from build123d import *

# Parameters (mm, degrees)
F1_DEPTH = 38.1
F2_R     = 10.16
F3_DEPTH = 35.56
F5_DEPTH = 19.05
F7_DEPTH = 18.796


with BuildPart() as f1:
    # F0 (on Top) → F1 (new body)
    with BuildSketch(Plane.XY):
        Polygon((-12.0983748909, -20.955), (12.0983748909, -20.955), (24.1967497817, 0), (12.0983748909, 20.955), (-12.0983748909, 20.955), (-24.1967497817, 0), align=None)
    extrude(amount=F1_DEPTH)

    # F2 (on face) → F3 (cut)
    with BuildSketch(Plane.XY.offset(38.1)):
        with Locations((-5.499261314, 9.525)):
            Circle(F2_R)
        with Locations((5.499261314, -9.525)):
            Circle(F2_R)
    extrude(amount=-F3_DEPTH, mode=Mode.SUBTRACT)

    # F4 (on face) → F5 (cut)
    with BuildSketch(Plane(origin=(0, 0, 0), x_dir=(1, 0, 0), z_dir=(0, 0, -1))):
        Polygon((-15.9478578107, 9.2075), (-18.1475623363, 10.4775), (-19.4175623363, 8.2777954744), (-17.8528578107, 5.9079432116), align=None)
        Polygon((-16.8775623363, 12.6772045256), (-18.1475623363, 10.4775), (-15.9478578107, 9.2075), (-14.0428578107, 12.5070567884), align=None)
    extrude(amount=-F5_DEPTH, mode=Mode.SUBTRACT)

    # F6 (on face) → F7 (join)
    with BuildSketch(Plane(origin=(0, 0, 0), x_dir=(1, 0, 0), z_dir=(0, 0, -1))):
        Polygon((-2.286, 20.955), (0, 20.955), (0, 23.241), (-3.429, 23.241), align=None)
        Polygon((0, 23.241), (0, 20.955), (2.286, 20.955), (3.429, 23.241), align=None)
    extrude(amount=-F7_DEPTH)


solid = f1.part
Check sheet for the modelled part. Datum: model origin and axes. Units: mm. A direction names the side the tool comes from. Coordinates: 2 decimals unless noted, no trailing zeros. Loops run counter-clockwise (first coordinate to the right, second up) from the corner with the lowest first, then second, coordinate; pieces in that order, holes last. Notation, with made-up numbers: (41.5, 69.5) -> (65.5, 69.5) arc R7 ccw to (65.5, 74.5) -> close; hole circle Ø3 at (12, 59). An arc over 180 degrees is marked (long way). Answer in a Markdown table with one row per item.
1. Access from +Z, -Z, +X, -X, +Y, -Y to the whole of each face (thin tool, end or side, straight path). Record for faces 5 (the face through (2.85, -22.08, 9.27)), 6 (the face through (15.2, -6.5, 20.6)), 7 (the face through (-17, -10, 19.05)), 8 (the face through (-18.646, -7.109, 9.392)).
Check values:
| item | result |
|---|---|
| face 5 | +Z, -Z, +X |
| face 6 | +Z |
| face 7 | -Z |
| face 8 | -Z, -Y |
2. Release check for a two-part mould opening along Y. For faces 1 (the face through (0, -1, 0)), 2 (the face through (0, -23.241, 9)), 3 (the face through (5, -9, 2.54)), 4 (the face through (18.232, 10.331, 18.783)) record: released by +Y, released by -Y, zero draft, split by the parting line, or undercut.
Check values:
| item | result |
|---|---|
| face 1 | zero draft |
| face 2 | released by -Y |
| face 3 | undercut |
| face 4 | released by +Y |
3. Sectioned sample at D-D, the plane z = 21.5. Record the boundary of the cut face in (x, y) (3 decimals).
Check values:
| item | result |
|---|---|
| outline | (-24.197, 0) -> (-12.098, -20.955) -> (12.098, -20.955) -> (24.197, 0) -> (12.098, 20.955) -> (-12.098, 20.955) -> close; hole circle Ø20.32 at (-5.499, 9.525); hole circle Ø20.32 at (5.499, -9.525) |
4. Material ranges on line 1 along Y through (x, z) = (1.5, 35.5) (1 decimal); line 2 along Y through (x, z) = (-6, 13) (3 decimals); line 3 along Z through (x, y) = (-18.5, -8.5), recorded low to high. Write a range as [from, to].
Check values:
| item | result |
|---|---|
| line 1 | y = [-21, -18.9], [-0.2, 2.2], [16.9, 21] |
| line 2 | y = [-20.955, -0.623], [19.673, 20.955] |
| line 3 | z = [19.05, 38.1] |
5. Sectioned sample at C-C, the plane y = 1.5. Record the boundary of the cut face in (x, z).
Check values:
| item | result |
|---|---|
| outline | (-23.33, 0) -> (23.33, 0) -> (23.33, 38.1) -> (0.73, 38.1) -> (0.73, 2.54) -> (-11.73, 2.54) -> (-11.73, 38.1) -> (-23.33, 38.1) -> close |
6. Sectioned sample at B-B, the plane x = -7.5. Record the boundary of the cut face in (y, z) (3 decimals).
Check values:
| item | result |
|---|---|
| outline | (-20.955, 0) -> (20.955, 0) -> (20.955, 38.1) -> (19.486, 38.1) -> (19.486, 2.54) -> (-0.436, 2.54) -> (-0.436, 38.1) -> (-20.955, 38.1) -> close |
7. Go/stop test with flat-tipped pins: pin 1 (2 mm diameter, centred on x = -5.5, z = 19, fed in from -Y) (3 decimals); pin 2 (1.6 mm diameter, centred on x = -17.5, y = -9, fed in from -Z); pin 3 (3 mm diameter, centred on x = -2, y = 4.5, fed in from +Z). Record where each tip stops, or that it passes through.
Check values:
| item | result |
|---|---|
| pin 1 | stops at y = -20.955 |
| pin 2 | stops at z = 19.05 |
| pin 3 | stops at z = 2.54 |
8. Sectioned sample at A-A, the plane z = 10.5. Record the boundary of the cut face in (x, y) (3 decimals).
Check values:
| item | result |
|---|---|
| outline | (-24.197, 0) -> (-19.418, -8.278) -> (-17.853, -5.908) -> (-14.043, -12.507) -> (-16.878, -12.677) -> (-12.098, -20.955) -> (-2.286, -20.955) -> (-3.429, -23.241) -> (3.429, -23.241) -> (2.286, -20.955) -> (12.098, -20.955) -> (24.197, 0) -> (12.098, 20.955) -> (-12.098, 20.955) -> close; hole circle Ø20.32 at (-5.499, 9.525); hole circle Ø20.32 at (5.499, -9.525) |
